Autodesk Inventor part; units mm, degrees
ref_plane "YZ Plane" through (0, 0, 0) normal (1, 0, 0) x (0, 1, 0)
ref_plane "XZ Plane" through (0, 0, 0) normal (0, 1, 0) x (-1, 0, 0)
ref_plane "XY Plane" through (0, 0, 0) normal (0, 0, 1) x (1, 0, 0)
ref_plane "Work Plane1" through (0, 0, 0) normal (0, 0, 1) x (1, 0, 0)
sketch "Sketch1" plane through (0, 0, 0) normal (0, 0, 1) x (1, 0, 0)
  line L0 (39.878985, 283.001047) -> (46.807188, 279.001047)
  line L1 (118.687297, 237.501047) -> (-32.001123, 324.501047)
  line L2 (118.687297, 237.501047) -> (112.687297, 227.108743)
  line L3 (-38.001123, 314.108743) -> (112.687297, 227.108743)
  line L4 (-32.001123, 324.501047) -> (-38.001123, 314.108743)
  line L5 (40.807188, 268.608743) -> (46.807188, 279.001047)
  line L6 (33.878985, 272.608743) -> (39.878985, 283.001047)
  line L7 (40.807188, 268.608743) -> (33.878985, 272.608743)
  circle A0 centre (68.259454, 214.654052) radius 27.5 construction
  line L8 (52.931544, 261.608743) -> (21.754629, 279.608743)
  line L9 (21.754629, 279.608743) -> (15.754629, 269.216438)
  line L10 (15.754629, 269.216438) -> (46.931544, 251.216438)
  line L11 (46.931544, 251.216438) -> (52.931544, 261.608743)
  point P0 (0, 0)
  dimension "d0" = 55
  dimension "d1" = 12
  dimension "d2" = 14
  dimension "d3" = 14
sketch "Sketch1 outline for Extrusion1" plane through (0, 0, 0) normal (0, 0, 1) x (1, 0, 0)
  line L0 (15.754629, 269.216438) -> (46.931544, 251.216438)
  line L1 (21.754629, 279.608743) -> (15.754629, 269.216438)
  line L2 (52.931544, 261.608743) -> (21.754629, 279.608743)
  line L3 (46.931544, 251.216438) -> (52.931544, 261.608743)
extrude "Extrusion1" add sketch "Sketch1 outline for Extrusion1" along normal blind 10
fillet "Fillet1" radius 6 2 edges at (15.7546, 269.2164, 5) (46.9315, 251.2164, 5)
sketch "Sketch2" plane through (0, 0, 10) normal (0, 0, 1) x (1, 0, 0)
  arc A0 (18.754629, 274.41259) -> (20.950782, 266.216438) centre (23.950782, 271.41259) ccw
  arc A1 (41.735391, 254.216438) -> (49.931544, 256.41259) centre (44.735391, 259.41259) ccw
  point P0 (0, 0)
hole "Hole1" at (23.950782, 271.41259, 10) at (44.735391, 259.41259, 10) direction (0, 0, -1) diameter 3.5 end through all countersink diameter 8 countersink angle 90
sketch "Sketch3" plane through (0, 0, 10) normal (0, 0, 1) x (1, 0, 0)
  line L0 (52.931544, 261.608743) -> (21.754629, 279.608743)
  line L1 (42.539239, 267.608743) -> (32.146934, 273.608743)
  line L2 (32.146934, 273.608743) -> (26.146934, 263.216438)
  line L3 (26.146934, 263.216438) -> (36.539239, 257.216438)
  line L4 (36.539239, 257.216438) -> (42.539239, 267.608743)
  line L5 (21.754629, 279.608743) -> (18.754629, 274.41259)
  line L6 (49.931544, 256.41259) -> (52.931544, 261.608743)
  point P0 (0, 0)
  dimension "d14" = 12
  dimension "d15" = 12
  dimension "d16" = 12
sketch "Sketch3 outline for Extrusion2" plane through (0, 0, 10) normal (0, 0, 1) x (1, 0, 0)
  line L0 (26.146934, 263.216438) -> (36.539239, 257.216438)
  line L1 (32.146934, 273.608743) -> (26.146934, 263.216438)
  line L2 (42.539239, 267.608743) -> (32.146934, 273.608743)
  line L3 (36.539239, 257.216438) -> (42.539239, 267.608743)
extrude "Extrusion2" add sketch "Sketch3 outline for Extrusion2" along normal blind 47
sketch "Sketch4" plane through (21.754629, 279.608743, 10) normal (0.5, 0.8660254, 0) x (0.8660254, -0.5, 0)
  circle A0 centre (18, -41) radius 4
  point P0 (120.96431, 10)
sketch "Sketch4 outline for Extrusion3" plane through (21.754629, 279.608743, 10) normal (0.5, 0.8660254, 0) x (0.8660254, -0.5, 0)
  circle A0 centre (18, -41) radius 4
extrude "Extrusion3" cut sketch "Sketch4 outline for Extrusion3" against normal through all
fillet "Fillet2" radius 6 2 edges at (39.5392, 262.4126, 57) (29.1469, 268.4126, 57)
fillet "Fillet3" radius 1 2 edges at (29.1469, 268.4126, 10) (39.5392, 262.4126, 10)
draft "FaceDraft1" angle 2 pull direction (0, 0, 1) faces at (37.48227, 270.528385, 23.009722) fixed edges at (37.343087, 270.608743, 0)
sketch "Sketch6" plane through (49.931544, 256.41259, 10) normal (0.8660254, -0.5, 0) x (0, 0, -1)
  line L0 (0, 0) -> (0, -6)
  line L1 (0, -6) -> (10, -6)
  line L2 (10, -6) -> (10, 0)
  line L3 (10, 0) -> (0, 0)
  line L4 (10, 0) -> (0, 0)
  line L5 (10, 0) -> (10, 6)
  line L6 (10, 6) -> (0, 5.650792)
  line L7 (0, 0) -> (0, 5.650792)
  line L8 (-1, -6) -> (0, -6)
  line L9 (0, -6) -> (-53.172101, -6)
  line L10 (-53.172101, -6) -> (-53.172101, 15.66156)
  line L11 (-53.172101, 15.66156) -> (0, 15.66156)
  line L12 (0, 15.66156) -> (0, -6)
  point P0 (10, -247.025589)
  point P1 (0, 5.650792)
sketch "Sketch6 outline for Extrusion4" plane through (49.931544, 256.41259, 10) normal (0.8660254, -0.5, 0) x (0, 0, -1)
  line L0 (0, 15.66156) -> (-53.172101, 15.66156)
  line L1 (0, 5.650792) -> (0, 15.66156)
  line L2 (0, 0) -> (0, 5.650792)
  line L3 (0, -6) -> (0, 0)
  line L4 (-1, -6) -> (0, -6)
  line L5 (-53.172101, -6) -> (-1, -6)
  line L6 (-53.172101, 15.66156) -> (-53.172101, -6)
extrude "Extrusion4" cut sketch "Sketch6 outline for Extrusion4" against normal through all
equation "\"d2\" = d3"
equation "\"d15\" = d16"
properties part number "backcover_clamp_mini"
Verification items for the finished model (mm, model axes). Round coordinates to 2 decimals unless told otherwise and drop trailing zeros. Order: outer loops, then holes, each group sorted by start corner. A loop starts at its lowest first (then second) coordinate and runs counter-clockwise, first axis right, second up.
1) Cross-section at D-D, the plane y = 276.75. Record the cut outline in (x, z), plus the area to 3 significant figures.
Geometry says:
outline: (20.1, 0) - (26.71, 0) - (26.01, 10) - (20.1, 10) - close
area: 62.5 mm2
2) Material ranges on line 1 (Y direction, x = 23, z = 3.5); line 2 (Y direction, x = 44.5, z = 4.5); line 3 (X direction, y = 258.5, z = 2), recorded low to high.
Geometry says:
line 1: y = 265.03 to 269.94, 272.88 to 278.75
line 2: y = 253.42 to 257.68, 261.15 to 266.3
line 3: x = 34.32 to 43.24, 46.23 to 51.14
3) Cross-section at A-A, the plane z = 9. Record the cut outline in (x, y), plus the area to 3 significant figures.
Geometry says:
outline: (18.75, 274.41) arc R6 ccw to (20.95, 266.22) - (41.74, 254.22) arc R6 ccw to (49.93, 256.41) - (52.77, 261.34) - (21.6, 279.34) - close; hole circle Ø6 at (23.95, 271.41); hole circle Ø6 at (44.74, 259.41)
area: 349 mm2
4) Depth check by flat-ended pin: pin 1 (4 mm diameter, centred on x = 44.74, y = 259.41, fed in from +Z); pin 2 (3 mm diameter, centred on y = 267.5, z = 5.5, fed in from +X); pin 3 (1 mm diameter, centred on y = 268.5, z = 4, fed in from -X); pin 4 (4.5 mm diameter, centred on x = 23.95, y = 271.41, fed in from -Z). Enter the tip coordinate at first touch or a pass-through.
Geometry says:
pin 1: stops at z = 8.01
pin 2: stops at x = 44.94
pin 3: stops at x = 18.46
pin 4: stops at z = 0
5) Draft check along X on faces 1 (the cylindrical face through (46.22, 253.6, 5.07)), 2 (the flat face through (20.276, 277.047, 4.93)), 3 (the conical face through (45.3, 257.6, 7.9)), 4 (the flat face through (51.41, 258.97, 4.93)). Enter one of: +X half, -X half, draft (parallel to the pull), parting line (faces both ways), or undercut.
Geometry says:
face 1: parting line
face 2: -X half
face 3: undercut
face 4: +X half
6) Cross-section at C-C, the plane x = 32.5. Record the cut outline in (y, z), plus the area to 3 significant figures.
Geometry says:
outline: (259.55, 0) - (273.4, 0) - (273, 10) - (259.55, 10) - close
area: 137 mm2
7) Cross-section at B-B, the plane z = 2.5. Record the cut outline in (x, y), plus the area to 3 significant figures.
Geometry says:
outline: (18.75, 274.41) arc R6 ccw to (20.95, 266.22) - (41.74, 254.22) arc R6 ccw to (49.93, 256.41) - (52.89, 261.53) - (21.71, 279.53) - close; hole circle Ø3.5 at (23.95, 271.41); hole circle Ø3.5 at (44.74, 259.41)
area: 394 mm2
